Geometry: final body of the model. Coordinates: model frame, mm. A direction names the side the tool comes from. Round coordinates to 2 decimals unless told otherwise and drop trailing zeros. Write each loop counter-clockwise with the first axis right and the second up, starting at its lowest first coordinate (ties: lowest second). Pieces come first, ordered by that corner, then holes. Notation, with made-up numbers: (-2, 7) - (16, 7) arc R13 cw to (16, 32) - close; hole circle Ø6 at (31.5, 22). An arc over 180 degrees is marked (long way). Write each question's results on one line, items separated by ' | '.
from build123d import *

# Parameters (mm, degrees)
BOSS_EXTRUDE1_DEPTH = 3
SKETCH3_R           = 15
CUT_EXTRUDE1_DEPTH  = 3
CUT_EXTRUDE3_DEPTH  = 3
SKETCH7_R           = 2.4
CUT_EXTRUDE4_DEPTH  = 3


with BuildPart() as part:
    # Sketch1 → Boss-Extrude1 (new body)
    with BuildSketch(Plane.XY):
        Polygon((-62.133450379, -27.758203286), (7.199328029, -67.670179411), (66.582879797, -14.064267615), (33.951154754, 58.977983998), (-45.599912202, 50.514666314), align=None)
    extrude(amount=BOSS_EXTRUDE1_DEPTH)

    # Sketch3 → Cut-Extrude1 (cut)
    with BuildSketch(Plane.XY.offset(3)):
        Circle(SKETCH3_R)
    extrude(amount=-CUT_EXTRUDE1_DEPTH, mode=Mode.SUBTRACT)

    # Sketch5 → Cut-Extrude3 (cut)
    with BuildSketch(Plane.XY.offset(3)):
        Polygon((28.177848363, 6.856300869), (33.166845379, 15.52289817), (35.766824569, 14.026199065), (30.777827554, 5.359601764), align=None)
        Polygon((41.177744315, -0.627194654), (46.166741331, 8.039402647), (48.766720521, 6.542703542), (43.777723505, -2.123893759), align=None)
        Polygon((10.821839491, -29.30678744), (5.832842475, -37.973384741), (3.232863285, -36.476685636), (8.221860301, -27.810088335), align=None)
        Polygon((23.821735443, -36.790282963), (18.832738427, -45.456880264), (16.232759237, -43.960181159), (21.221756252, -35.293583858), align=None)
    extrude(amount=-CUT_EXTRUDE3_DEPTH, mode=Mode.SUBTRACT)

    # Sketch7 → Cut-Extrude4 (cut)
    with BuildSketch(Plane(origin=(0, 0, 0), x_dir=(-1, 0, 0), z_dir=(0, 0, -1))):
        with Locations((-25.78312697, -14.842266122)):
            Circle(SKETCH7_R)
    extrude(amount=-CUT_EXTRUDE4_DEPTH, mode=Mode.SUBTRACT)


solid = part.part
Q1. Ray query, line 1 along X through (y, z) = (-1, 0.9); line 2 along X through (y, z) = (-8, 0.9); line 3 along Y through (x, z) = (0, 0.8). Return the intervals inside material, ascending.
Answer block:
line 1: -56.48 to -14.97, 14.97 to 41.83, 44.42 to 60.75 | line 2: -57.96 to -12.69, 12.69 to 63.87 | line 3: -63.53 to -15, 15 to 55.37
Q2. Section query B-B, the plane z = 1.2. Return loops of the section in (x, y), plus the area to 3 significant figures.
Answer block:
outline: (-62.13, -27.76) - (7.2, -67.67) - (66.58, -14.06) - (33.95, 58.98) - (-45.6, 50.51) - close; hole circle Ø30 at (0, 0); hole (3.23, -36.48) - (5.83, -37.97) - (10.82, -29.31) - (8.22, -27.81) - close; hole (16.23, -43.96) - (18.83, -45.46) - (23.82, -36.79) - (21.22, -35.29) - close; hole circle Ø4.8 at (25.78, -14.84); hole (28.18, 6.86) - (30.78, 5.36) - (35.77, 14.03) - (33.17, 15.52) - close; hole (41.18, -0.63) - (43.78, -2.12) - (48.77, 6.54) - (46.17, 8.04) - close | area: 10,200 mm2
Q3. Section query D-D, the plane y = 38. Return loops of the section in (x, z), plus the area to 3 significant figures.
Answer block:
outline: (-48.24, 0) - (43.32, 0) - (43.32, 3) - (-48.24, 3) - close | area: 275 mm2
Q4. Access query for faces 1 (the flat face through (16, -3, 3)), 2 (the flat face through (8.36, -33.58, 1.52)). Directions: +Z, -Z, +X, -X, +Y, -Y. A direction counts if a zero-diameter tool reaches every point of the face in a straight line with its end or side. Return the directions, or none.
Answer block:
face 1: +Z, +X, -X, +Y, -Y | face 2: +Z, -Z
Q5. Mould query, pull axis Y, two halves, no side actions, for faces 3 (the flat face through (36.48, -41.24, 1.48)), 4 (the flat face through (16, -3, 0)), 5 (the flat face through (33.307, 9.754, 1.521)). Classes: pulls with the +Y half, pulls with the -Y half, needs draft (parallel to the pull), parting line crosses it, or undercut.
Answer block:
face 3: pulls with the -Y half | face 4: needs draft | face 5: undercut
Q6. Pin query (flat end, axial travel): pin 1 (1.5 mm diameter, centred on x = 29.5, z = 1, fed in from +Y); pin 2 (1.5 mm diameter, centred on y = -46, z = 2.5, fed in from +X). Return the tip coordinate at first contact, or that it passes through.
Answer block:
pin 1: y = 58.58 | pin 2: x = 32.04
Q7. Section query A-A, the plane x = -10.5. Return loops of the section in (y, z).
Answer block:
outline: (-57.48, 0) - (-10.71, 0) - (-10.71, 3) - (-57.48, 3) - close; (10.71, 0) - (54.25, 0) - (54.25, 3) - (10.71, 3) - close
Q8. Section query C-C, the plane y = -9.5. Return loops of the section in (x, z).
Answer block:
outline: (-58.28, 0) - (-11.61, 0) - (-11.61, 3) - (-58.28, 3) - close; (11.61, 0) - (64.54, 0) - (64.54, 3) - (11.61, 3) - close
